```python
from build123d import *

# Parameters (mm, degrees)
MODEL_R                 = 1.5
SALIENTE_EXTRUIR1_DEPTH = 3


with BuildPart() as part:
    # Model → Saliente-Extruir1 (new body)
    with BuildSketch(Plane.XY):
        with BuildLine():
            Line((213.25077615, 89.428489513), (213.25077615, 188.428489513))
            ThreePointArc((213.25077615, 188.428489513), (208.75077615, 192.928489513), (204.25077615, 188.428489513))
            Line((204.25077615, 188.428489513), (204.25077615, 89.428489513))
            ThreePointArc((204.25077615, 89.428489513), (208.75077615, 84.928489513), (213.25077615, 89.428489513))
        make_face()
        with Locations((208.75077615, 179.428489513)):
            Circle(MODEL_R, mode=Mode.SUBTRACT)
        with Locations((208.75077615, 188.428489513)):
            Circle(MODEL_R, mode=Mode.SUBTRACT)
        with Locations((208.75077615, 152.428489513)):
            Circle(MODEL_R, mode=Mode.SUBTRACT)
        with Locations((208.75077615, 161.428489513)):
            Circle(MODEL_R, mode=Mode.SUBTRACT)
        with Locations((208.75077615, 170.428489513)):
            Circle(MODEL_R, mode=Mode.SUBTRACT)
        with Locations((208.75077615, 143.428489513)):
            Circle(MODEL_R, mode=Mode.SUBTRACT)
        with Locations((208.75077615, 116.428489513)):
            Circle(MODEL_R, mode=Mode.SUBTRACT)
        with Locations((208.75077615, 125.428489513)):
            Circle(MODEL_R, mode=Mode.SUBTRACT)
        with Locations((208.75077615, 134.428489513)):
            Circle(MODEL_R, mode=Mode.SUBTRACT)
        with Locations((208.75077615, 89.428489513)):
            Circle(MODEL_R, mode=Mode.SUBTRACT)
        with Locations((208.75077615, 98.428489513)):
            Circle(MODEL_R, mode=Mode.SUBTRACT)
        with Locations((208.75077615, 107.428489513)):
            Circle(MODEL_R, mode=Mode.SUBTRACT)
    extrude(amount=SALIENTE_EXTRUIR1_DEPTH)


solid = part.part
```
CAD build for the part. Positions are in the model's coordinates, mm. Give positions to 0.01 mm unless a question says otherwise; leave off trailing zeros. Loops run counter-clockwise (first coordinate to the right, second up) from the corner with the lowest first, then second, coordinate; pieces in that order, holes last. Notation, with made-up numbers: (60, -14) - (84, -14) arc R16 cw to (84, 0) - close; hole circle Ø7 at (-35.5, -5.5). An arc over 180 degrees is marked (long way). Put each result on its own line as item: value.
Q1. Slice it at A-A (z = 1.6). Give the number of separate pieces and of enclosed holes in the cut face, plus the area to 3 significant figures.
Filled in:
separate pieces: 1
enclosed holes: 12
area: 870 mm²
Q2. Mould opens along X. For faces 1 (the face through (208.85, 192.927, 1.479)), 2 (the face through (207.252, 125.494, 1.479)), 3 (the face through (209, 140, 3)) say: pulls with the +X half, pulls with the -X half, needs draft (parallel to the pull), parting line crosses it, or undercut.
Filled in:
face 1: parting line crosses it
face 2: undercut
face 3: needs draft
Q3. Probe line 1 along X through (y, z) = (98, 1.8); line 2 along X through (y, z) = (89, 1); line 3 along Y through (x, z) = (205.25, 2.3). List the from-to ranges inside material, lowest first.
Filled in:
line 1: x = 204.25 to 207.31, 210.19 to 213.25
line 2: x = 204.27 to 207.31, 210.19 to 213.23
line 3: y = 86.6 to 191.26
Q4. Slice it at B-B (x = 212). Give the cut face in (y, z).
Filled in:
outline: (86.32, 0) - (191.54, 0) - (191.54, 3) - (86.32, 3) - close
